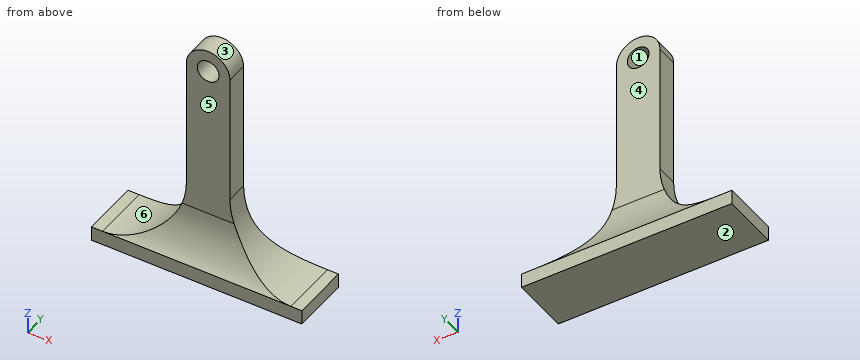
```python
from build123d import *

# Parameters (mm, degrees)
SKETCH1_W           = 29
SKETCH1_H           = 8
BOSS_EXTRUDE1_DEPTH = 2
SKETCH2_R           = 1.5
BOSS_EXTRUDE2_DEPTH = 1.5
FILLET1_R           = 10


with BuildPart() as part:
    # Sketch1 → Boss-Extrude1 (new body)
    with BuildSketch(Plane.XY):
        Rectangle(SKETCH1_W, SKETCH1_H)
    extrude(amount=BOSS_EXTRUDE1_DEPTH)

    # Sketch2 → Boss-Extrude2 (add, symmetric)
    with BuildSketch(Plane(origin=(0, 0, 0), x_dir=(1, 0, 0), z_dir=(0, 1, 0))):
        with BuildLine():
            Line((-3, -2), (3, -2))
            Line((3, -2), (3, -30))
            ThreePointArc((3, -30), (0, -33), (-3, -30))
            Line((-3, -30), (-3, -2))
        make_face()
        with Locations(Location((0, -30, 0), (0, 0, 270))):
            Circle(SKETCH2_R, mode=Mode.SUBTRACT)
    extrude(amount=BOSS_EXTRUDE2_DEPTH, both=True)

    # Fillet1
    # the kernel refuses this fillet: 10 mm, written as the material it adds along each edge
    with BuildSketch(Plane(origin=(-3, 1.5, 2), x_dir=(0, 1, 0), z_dir=(1, 0, 0))) as fillet1_piece_1:
        with BuildLine():
            CenterArc((10, 6.614378278), FILLET1_R, 180, 41.409622109)
            Line((0, 6.614378278), (-0.2, 6.614378278))
            Line((-0.2, 6.614378278), (-0.2, 0))
            Line((-0.2, 0), (0, -0.2))
            ThreePointArc((0, -0.2), (1.25, -0.2), (2.35, -0.132287566))
            Line((2.35, -0.132287566), (2.5, 0))
        make_face()
    extrude(amount=6)
    with BuildSketch(Plane(origin=(-3, -1.5, 2), x_dir=(-1, 0, 0), z_dir=(0, 1, 0)), Plane(origin=(3, 1.5, 2), x_dir=(1, 0, 0), z_dir=(0, -1, 0))) as fillet1_piece_2:
        with BuildLine():
            CenterArc((FILLET1_R, FILLET1_R), FILLET1_R, 180, 90)
            Line((0, FILLET1_R), (-FILLET1_R * 0.02, FILLET1_R))
            Line((-FILLET1_R * 0.02, FILLET1_R), (-FILLET1_R * 0.02, -FILLET1_R * 0.02))
            Line((-FILLET1_R * 0.02, -FILLET1_R * 0.02), (FILLET1_R, -FILLET1_R * 0.02))
            Line((FILLET1_R, -FILLET1_R * 0.02), (FILLET1_R, 0))
        make_face()
    extrude(amount=3)
    with BuildSketch(Plane(origin=(-3, -1.5, 2), x_dir=(0, -1, 0), z_dir=(1, 0, 0))) as fillet1_piece_3:
        with BuildLine():
            CenterArc((10, -6.614378278), FILLET1_R, 138.590377891, 41.409622109)
            Line((0, -6.614378278), (-0.2, -6.614378278))
            Line((-0.2, -6.614378278), (-0.2, 0))
            Line((-0.2, 0), (0, 0.2))
            ThreePointArc((0, 0.2), (1.25, 0.2), (2.35, 0.132287566))
            Line((2.35, 0.132287566), (2.5, 0))
        make_face()
    extrude(amount=6)
    with BuildSketch(Plane(origin=(-19.535945694, 1.5, 2), x_dir=(0, 1, 0), z_dir=(1, 0, 0))) as fillet1_piece_4a_section:
        with BuildLine():
            CenterArc((10, 6.614378278), FILLET1_R, 180, 41.409622109)
            Line((0, 6.614378278), (-0.2, 6.614378278))
            Line((-0.2, 6.614378278), (-0.2, 0))
            Line((-0.2, 0), (0, -0.2))
            ThreePointArc((0, -0.2), (1.25, -0.2), (2.35, -0.132287566))
            Line((2.35, -0.132287566), (2.5, 0))
        make_face()
    fillet1_piece_4a = extrude(amount=22.535945694, mode=Mode.PRIVATE)
    fillet1_piece_4a = split(fillet1_piece_4a, bisect_by=Plane(origin=(-14.5, 2.097749904, 3.814075663), z_dir=(1, 0, 0)), keep=Keep.TOP, mode=Mode.PRIVATE)
    fillet1_piece_4a = split(fillet1_piece_4a, bisect_by=Plane(origin=(-3, 2.097749904, 3.814075663), z_dir=(-1, 0, 0)), keep=Keep.TOP, mode=Mode.PRIVATE)
    with BuildSketch(Plane(origin=(-3, -1.5, 2), x_dir=(-1, 0, 0), z_dir=(0, 1, 0))) as fillet1_piece_4b_section:
        with BuildLine():
            CenterArc((FILLET1_R, FILLET1_R), FILLET1_R, 180, 90)
            Line((0, FILLET1_R), (-FILLET1_R * 0.02, FILLET1_R))
            Line((-FILLET1_R * 0.02, FILLET1_R), (-FILLET1_R * 0.02, -FILLET1_R * 0.02))
            Line((-FILLET1_R * 0.02, -FILLET1_R * 0.02), (FILLET1_R, -FILLET1_R * 0.02))
            Line((FILLET1_R, -FILLET1_R * 0.02), (FILLET1_R, 0))
        make_face()
    fillet1_piece_4b = extrude(amount=28, mode=Mode.PRIVATE)
    fillet1_piece_4b = split(fillet1_piece_4b, bisect_by=Plane(origin=(-5.263951143, 4, 4.263951143), z_dir=(0, -1, 0)), keep=Keep.TOP, mode=Mode.PRIVATE)
    fillet1_piece_4b = split(fillet1_piece_4b, bisect_by=Plane(origin=(-5.263951143, 1.5, 4.263951143), z_dir=(0, 1, 0)), keep=Keep.TOP, mode=Mode.PRIVATE)
    fillet1_piece_4 = fillet1_piece_4a & fillet1_piece_4b
    add(fillet1_piece_4)
    with BuildSketch(Plane(origin=(3, 26.5, 2), x_dir=(1, 0, 0), z_dir=(0, -1, 0))) as fillet1_piece_5a_section:
        with BuildLine():
            CenterArc((FILLET1_R, FILLET1_R), FILLET1_R, 180, 90)
            Line((0, FILLET1_R), (-FILLET1_R * 0.02, FILLET1_R))
            Line((-FILLET1_R * 0.02, FILLET1_R), (-FILLET1_R * 0.02, -FILLET1_R * 0.02))
            Line((-FILLET1_R * 0.02, -FILLET1_R * 0.02), (FILLET1_R, -FILLET1_R * 0.02))
            Line((FILLET1_R, -FILLET1_R * 0.02), (FILLET1_R, 0))
        make_face()
    fillet1_piece_5a = extrude(amount=28, mode=Mode.PRIVATE)
    fillet1_piece_5a = split(fillet1_piece_5a, bisect_by=Plane(origin=(5.263951143, 4, 4.263951143), z_dir=(0, -1, 0)), keep=Keep.TOP, mode=Mode.PRIVATE)
    fillet1_piece_5a = split(fillet1_piece_5a, bisect_by=Plane(origin=(5.263951143, 1.5, 4.263951143), z_dir=(0, 1, 0)), keep=Keep.TOP, mode=Mode.PRIVATE)
    with BuildSketch(Plane(origin=(-3, 1.5, 2), x_dir=(0, 1, 0), z_dir=(1, 0, 0))) as fillet1_piece_5b_section:
        with BuildLine():
            CenterArc((10, 6.614378278), FILLET1_R, 180, 41.409622109)
            Line((0, 6.614378278), (-0.2, 6.614378278))
            Line((-0.2, 6.614378278), (-0.2, 0))
            Line((-0.2, 0), (0, -0.2))
            ThreePointArc((0, -0.2), (1.25, -0.2), (2.35, -0.132287566))
            Line((2.35, -0.132287566), (2.5, 0))
        make_face()
    fillet1_piece_5b = extrude(amount=22.535945694, mode=Mode.PRIVATE)
    fillet1_piece_5b = split(fillet1_piece_5b, bisect_by=Plane(origin=(14.5, 2.097749904, 3.814075663), z_dir=(-1, 0, 0)), keep=Keep.TOP, mode=Mode.PRIVATE)
    fillet1_piece_5b = split(fillet1_piece_5b, bisect_by=Plane(origin=(3, 2.097749904, 3.814075663), z_dir=(1, 0, 0)), keep=Keep.TOP, mode=Mode.PRIVATE)
    fillet1_piece_5 = fillet1_piece_5a & fillet1_piece_5b
    add(fillet1_piece_5)
    with BuildSketch(Plane(origin=(-19.535945694, -1.5, 2), x_dir=(0, -1, 0), z_dir=(1, 0, 0))) as fillet1_piece_6a_section:
        with BuildLine():
            CenterArc((10, -6.614378278), FILLET1_R, 138.590377891, 41.409622109)
            Line((0, -6.614378278), (-0.2, -6.614378278))
            Line((-0.2, -6.614378278), (-0.2, 0))
            Line((-0.2, 0), (0, 0.2))
            ThreePointArc((0, 0.2), (1.25, 0.2), (2.35, 0.132287566))
            Line((2.35, 0.132287566), (2.5, 0))
        make_face()
    fillet1_piece_6a = extrude(amount=22.535945694, mode=Mode.PRIVATE)
    fillet1_piece_6a = split(fillet1_piece_6a, bisect_by=Plane(origin=(-14.5, -2.097749904, 3.814075663), z_dir=(1, 0, 0)), keep=Keep.TOP, mode=Mode.PRIVATE)
    fillet1_piece_6a = split(fillet1_piece_6a, bisect_by=Plane(origin=(-3, -2.097749904, 3.814075663), z_dir=(-1, 0, 0)), keep=Keep.TOP, mode=Mode.PRIVATE)
    with BuildSketch(Plane(origin=(-3, -26.5, 2), x_dir=(-1, 0, 0), z_dir=(0, 1, 0))) as fillet1_piece_6b_section:
        with BuildLine():
            CenterArc((FILLET1_R, FILLET1_R), FILLET1_R, 180, 90)
            Line((0, FILLET1_R), (-FILLET1_R * 0.02, FILLET1_R))
            Line((-FILLET1_R * 0.02, FILLET1_R), (-FILLET1_R * 0.02, -FILLET1_R * 0.02))
            Line((-FILLET1_R * 0.02, -FILLET1_R * 0.02), (FILLET1_R, -FILLET1_R * 0.02))
            Line((FILLET1_R, -FILLET1_R * 0.02), (FILLET1_R, 0))
        make_face()
    fillet1_piece_6b = extrude(amount=28, mode=Mode.PRIVATE)
    fillet1_piece_6b = split(fillet1_piece_6b, bisect_by=Plane(origin=(-5.263951143, -4, 4.263951143), z_dir=(0, 1, 0)), keep=Keep.TOP, mode=Mode.PRIVATE)
    fillet1_piece_6b = split(fillet1_piece_6b, bisect_by=Plane(origin=(-5.263951143, -1.5, 4.263951143), z_dir=(0, -1, 0)), keep=Keep.TOP, mode=Mode.PRIVATE)
    fillet1_piece_6 = fillet1_piece_6a & fillet1_piece_6b
    add(fillet1_piece_6)
    with BuildSketch(Plane(origin=(-3, -1.5, 2), x_dir=(0, -1, 0), z_dir=(1, 0, 0))) as fillet1_piece_7a_section:
        with BuildLine():
            CenterArc((10, -6.614378278), FILLET1_R, 138.590377891, 41.409622109)
            Line((0, -6.614378278), (-0.2, -6.614378278))
            Line((-0.2, -6.614378278), (-0.2, 0))
            Line((-0.2, 0), (0, 0.2))
            ThreePointArc((0, 0.2), (1.25, 0.2), (2.35, 0.132287566))
            Line((2.35, 0.132287566), (2.5, 0))
        make_face()
    fillet1_piece_7a = extrude(amount=22.535945694, mode=Mode.PRIVATE)
    fillet1_piece_7a = split(fillet1_piece_7a, bisect_by=Plane(origin=(14.5, -2.097749904, 3.814075663), z_dir=(-1, 0, 0)), keep=Keep.TOP, mode=Mode.PRIVATE)
    fillet1_piece_7a = split(fillet1_piece_7a, bisect_by=Plane(origin=(3, -2.097749904, 3.814075663), z_dir=(1, 0, 0)), keep=Keep.TOP, mode=Mode.PRIVATE)
    with BuildSketch(Plane(origin=(3, 1.5, 2), x_dir=(1, 0, 0), z_dir=(0, -1, 0))) as fillet1_piece_7b_section:
        with BuildLine():
            CenterArc((FILLET1_R, FILLET1_R), FILLET1_R, 180, 90)
            Line((0, FILLET1_R), (-FILLET1_R * 0.02, FILLET1_R))
            Line((-FILLET1_R * 0.02, FILLET1_R), (-FILLET1_R * 0.02, -FILLET1_R * 0.02))
            Line((-FILLET1_R * 0.02, -FILLET1_R * 0.02), (FILLET1_R, -FILLET1_R * 0.02))
            Line((FILLET1_R, -FILLET1_R * 0.02), (FILLET1_R, 0))
        make_face()
    fillet1_piece_7b = extrude(amount=28, mode=Mode.PRIVATE)
    fillet1_piece_7b = split(fillet1_piece_7b, bisect_by=Plane(origin=(5.263951143, -4, 4.263951143), z_dir=(0, 1, 0)), keep=Keep.TOP, mode=Mode.PRIVATE)
    fillet1_piece_7b = split(fillet1_piece_7b, bisect_by=Plane(origin=(5.263951143, -1.5, 4.263951143), z_dir=(0, -1, 0)), keep=Keep.TOP, mode=Mode.PRIVATE)
    fillet1_piece_7 = fillet1_piece_7a & fillet1_piece_7b
    add(fillet1_piece_7)


solid = part.part
```
The model under review builds one solid part; all positions refer to its coordinate system, in mm. Face numbers are marked on the shaded views. A direction names the side the tool comes from. Round coordinates to 2 decimals unless told otherwise and drop trailing zeros. Order: outer loops, then holes, each group sorted by start corner. A loop starts at its lowest first (then second) coordinate and runs counter-clockwise, first axis right, second up. Notation, with made-up numbers: (32, 67.5) - (37, 67.5) arc R33 cw to (37, 100.5) - close; hole circle Ø4 at (23.25, 36.25). An arc over 180 degrees is marked (long way). Answer in a Markdown table with one row per item.
(1) Take a section at D-D on y = 3.5. Write out the cut boundary in (x, z), plus the area to 3 significant figures.
Result set:
| item | result |
|---|---|
| outline | (-14.5, 0) - (14.5, 0) - (14.5, 2) - (13, 2) arc R10 cw to (9.55, 2.61) - (-9.55, 2.61) arc R10 cw to (-13, 2) - (-14.5, 2) - close |
| area | 71.1 mm2 |
(2) Take a section at A-A on x = 0. Write out the cut boundary in (y, z).
Result set:
| item | result |
|---|---|
| outline | (-4, 0) - (4, 0) - (4, 2) arc R10 cw to (1.5, 8.61) - (1.5, 28.5) - (-1.5, 28.5) - (-1.5, 8.61) arc R10 cw to (-4, 2) - close; (-1.5, 31.5) - (1.5, 31.5) - (1.5, 33) - (-1.5, 33) - close |
(3) Machinability: for the marked faces 5 and 6, which of the approach directions +Z, -Z, +X, -X, +Y, -Y give a long, thin tool a straight path to every point of the face, cutting with its end or side? Answer none if there is none.
Result set:
| item | result |
|---|---|
| face 5 | +Z, +X, -X, -Y |
| face 6 | +Z, -X, +Y, -Y |
(4) Mouldability with a two-part tool opening along Z and no side actions: class the marked faces 1, 2, 3 and 4 as released by +Z, released by -Z, zero draft, split by the parting line, or undercut.
Result set:
| item | result |
|---|---|
| face 1 | undercut |
| face 2 | released by -Z |
| face 3 | released by +Z |
| face 4 | zero draft |
(5) Take a section at B-B on y = 0.5. Write out the cut boundary in (x, z).
Result set:
| item | result |
|---|---|
| outline | (-14.5, 0) - (14.5, 0) - (14.5, 2) - (13, 2) arc R10 cw to (3, 12) - (3, 30) arc R3 ccw to (-3, 30) - (-3, 12) arc R10 cw to (-13, 2) - (-14.5, 2) - close; hole circle Ø3 at (0, 30) |
(6) Take a section at C-C on z = 19. Write out the cut boundary in (x, y).
Result set:
| item | result |
|---|---|
| outline | (-3, -1.5) - (3, -1.5) - (3, 1.5) - (-3, 1.5) - close |
(7) Clearance check with flat-ended pins moving along their axes: P1, Ø0.9, axis at y = 0, z = 25, coming from the +X side; P2, Ø5.5, axis at x = 0.5, z = 18.5, coming from the -Y side; P3, Ø0.9, axis at y = -0.5, z = 19, coming from the -X side. State where each tip first meets the part, or that it passes through.
Result set:
| item | result |
|---|---|
| P1 | stops at x = 3 |
| P2 | stops at y = -1.5 |
| P3 | stops at x = -3 |
(8) For line 1 (X direction, y = 0.1, z = 30); line 2 (X direction, y = 0.25, z = 27); line 3 (Y direction, x = -2.25, z = 2.5), list the stretches that pass through material, from the lowest coordinate up. Write a range as from..to.
Result set:
| item | result |
|---|---|
| line 1 | x = -3..-1.5, 1.5..3 |
| line 2 | x = -3..3 |
| line 3 | y = -3.59..3.59 |
